The listing builds one solid part. Answer for the finished solid, in the listing's coordinates (mm). A direction names the side the tool comes from. Round coordinates to 2 decimals unless told otherwise and drop trailing zeros. Write each loop counter-clockwise with the first axis right and the second up, starting at its lowest first coordinate (ties: lowest second). Pieces come first, ordered by that corner, then holes. Notation, with made-up numbers: (48, 15.5) - (92, 15.5) arc R36 cw to (92, 49.5) - close; hole circle Ø2 at (-17, 85). An arc over 180 degrees is marked (long way). Return JSON: item names as keys, results as strings. Group by question number.
(1) Find the intervals of material crossed by line 1 along Y through (x, z) = (61.5, 58); line 2 along X through (y, z) = (19.45, 48); line 3 along Z through (x, y) = (61.75, 22.75), in increasing order. Write a range as [from, to].
(2) Determine the mould class of faces 4 (the flat face through (66, 17.5, 48)), 5 (the cylindrical face through (66.3, 19.27, 68.07)), 6 (the flat face through (55, 17, 72)) for opening direction X: +X half, -X half, draft (parallel to the pull), parting line (faces both ways), or undercut.
(3) Section C-C, the plane x = 54.25 is taken. Write down the section's boundary in (y, z), then the cut area to 3 significant figures.
(4) Each of these flat-tipped pins is pushed along its axis until it touches: pin 1 (4 mm diameter, centred on y = 15, z = 44.5, fed in from -X); pin 2 (8 mm diameter, centred on x = 61, y = 30.5, fed in from -Z); pin 3 (4.5 mm diameter, centred on x = 68, z = 49, fed in from -Y). Where does it stop, or does it pass through?
(5) Section D-D, the plane y = 31.75 is taken. Write down the section's boundary in (x, z).
(6) Section A-A, the plane y = 29 is taken. Write down the section's boundary in (x, z), then the cut area to 3 significant figures.
(7) Which of the six approach directions +Z, -Z, +X, -X, +Y, -Y give full straight-line access (tool end or side, diameter ignored) to faces 1 (the cylindrical face through (62.5, 27.145, 56.817)), 2 (the cylindrical face through (63.14, 27.1, 47.48)), 3 (the cylindrical face through (58.017, 24.76, 47.521))?
(8) Section B-B, the plane z = 59 is taken. Write down the section's boundary in (x, y), then the cut area to 3 significant figures.
```python
from build123d import *

# Parameters (mm, degrees)
BOX001027045206_W       = 8
BOX001027045206_H       = 6
BOX001027045206_DEPTH   = 10
CYLINDER272_R           = 2.2
CYLINDER272_DEPTH       = 30
CYLINDER271_R           = 2.2
CYLINDER271_DEPTH       = 30
CYLINDER271_PITCH_ANGLE = 90
CYLINDER270_R           = 1.7
CYLINDER270_DEPTH       = 30
CYLINDER270_PITCH_ANGLE = 90
BOX001027045200_W       = 10
BOX001027045200_H       = 9
BOX001027045200_DEPTH   = 10
CHAMFER015_SIZE         = 2
CHAMFER016_SIZE         = 2
FILLET046_R             = 3
CYLINDER045_R           = 1.9
CYLINDER045_DEPTH       = 200
BOX030_W                = 5.5
BOX030_H                = 10
BOX030_DEPTH            = 2.5
CYLINDER048_R           = 5.5
CYLINDER048_DEPTH       = 10
CYLINDER048_ROLL_ANGLE  = 90
CYLINDER050_R           = 5.5
CYLINDER050_DEPTH       = 10
CYLINDER050_ROLL_ANGLE  = 90
CYLINDER052_R           = 1.7
CYLINDER052_DEPTH       = 30
CYLINDER052_ROLL_ANGLE  = 90
CYLINDER053_R           = 1.7
CYLINDER053_DEPTH       = 30
CYLINDER053_ROLL_ANGLE  = 90
CYLINDER054_R           = 1.7
CYLINDER054_DEPTH       = 30
CYLINDER054_ROLL_ANGLE  = 90
CYLINDER047_R           = 5.5
CYLINDER047_DEPTH       = 10
CYLINDER047_ROLL_ANGLE  = 90
CYLINDER049_R           = 3
CYLINDER049_DEPTH       = 10
CYLINDER049_ROLL_ANGLE  = 90
CYLINDER051_R           = 3
CYLINDER051_DEPTH       = 10
CYLINDER051_ROLL_ANGLE  = 90
CYLINDER046_R           = 3
CYLINDER046_DEPTH       = 10
CYLINDER046_ROLL_ANGLE  = 90
BOX028_W                = 13
BOX028_H                = 8.5
BOX028_DEPTH            = 40
CHAMFER006_SIZE         = 2.5
CYLINDER273_R           = 2
CYLINDER273_DEPTH       = 10
CYLINDER273_PITCH_ANGLE = 90
BOX001027045201_W       = 3
BOX001027045201_H       = 8
BOX001027045201_DEPTH   = 8
FILLET047_R             = 3
CUT247_PITCH_ANGLE      = 90
CUT247_PLACEMENT_ANGLE  = 90


with BuildPart() as cube252:
    # Box001027045206 → Box001027045206 (new body)
    with BuildSketch(Plane(origin=(59.1, 20, 53), x_dir=(1, 0, 0), z_dir=(0, 0, 1))):
        with Locations((4, 3)):
            Rectangle(BOX001027045206_W, BOX001027045206_H)
    extrude(amount=BOX001027045206_DEPTH)


with BuildPart() as cylinder288:
    # Cylinder272 → Cylinder272 (new body)
    with BuildSketch(Plane(origin=(79.5, 5, 48), x_dir=(1, 0, 0), z_dir=(0, 0, 1))):
        Circle(CYLINDER272_R)
    extrude(amount=CYLINDER272_DEPTH)


with BuildPart() as cylinder287:
    # Cylinder271 → Cylinder271 (new body)
    with BuildSketch(Plane.XY):
        Circle(CYLINDER271_R)
    extrude(amount=CYLINDER271_DEPTH)


with BuildPart() as cylinder287_1:
    # Cylinder271 pitch: moved
    add(cylinder287.part.rotate(Axis((0, 0, 0), (0, 1, 0)), CYLINDER271_PITCH_ANGLE))


with BuildPart() as cylinder287_2:
    # Cylinder271 placement: moved
    add(cylinder287_1.part.moved(Location((74, 5, 58))))


with BuildPart() as cylinder286:
    # Cylinder270 → Cylinder270 (new body)
    with BuildSketch(Plane.XY):
        Circle(CYLINDER270_R)
    extrude(amount=CYLINDER270_DEPTH)


with BuildPart() as cylinder286_1:
    # Cylinder270 pitch: moved
    add(cylinder286.part.rotate(Axis((0, 0, 0), (0, 1, 0)), CYLINDER270_PITCH_ANGLE))


with BuildPart() as cylinder286_2:
    # Cylinder270 placement: moved
    add(cylinder286_1.part.moved(Location((57, 5, 58))))


with BuildPart() as led_pt_holder001:
    # Box001027045200 → Box001027045200 (new body)
    with BuildSketch(Plane(origin=(71, 1, 53), x_dir=(1, 0, 0), z_dir=(0, 0, 1))):
        with Locations((5, 4.5)):
            Rectangle(BOX001027045200_W, BOX001027045200_H)
    extrude(amount=BOX001027045200_DEPTH)

    # Chamfer015
    chamfer015_edges = [led_pt_holder001.edges().sort_by_distance(p)[0] for p in [
        (71, 10, 58),
    ]]
    chamfer(chamfer015_edges, length=CHAMFER015_SIZE)


with BuildPart() as led_pt_holder001_1:
    # Chamfer015 placement: moved
    add(led_pt_holder001.part.moved(Location((-1.5, 0, 0))))

    # Chamfer016
    chamfer016_edges = [led_pt_holder001_1.edges().sort_by_distance(p)[0] for p in [
        (69.5, 4.5, 63),
        (69.5, 4.5, 53),
    ]]
    chamfer(chamfer016_edges, length=CHAMFER016_SIZE)

    # Cut242: cut Cylinder286
    add(cylinder286_2.part, mode=Mode.SUBTRACT)

    # Cut243: cut Cylinder287
    add(cylinder287_2.part, mode=Mode.SUBTRACT)

    # Fillet046
    fillet046_edges = [led_pt_holder001_1.edges().sort_by_distance(p)[0] for p in [
        (69.5, 4.5, 55),
        (69.5, 4.5, 61),
    ]]
    fillet(fillet046_edges, radius=FILLET046_R)

    # Cut245: cut Cylinder288
    add(cylinder288.part, mode=Mode.SUBTRACT)


with BuildPart() as part_mirroring015:
    # Part__Mirroring015: instance of led-pt-holder001
    add(led_pt_holder001_1.part.mirror(Plane(origin=(60, 0, 0), x_dir=(0, -1, 0), z_dir=(1, 0, 0))))


with BuildPart() as part_mirroring015_1:
    # Part__Mirroring015 placement: moved
    add(part_mirroring015.part.moved(Location((18.6, 0, 0))))


with BuildPart() as pt_holder:
    # Part__Mirroring019: instance of Part__Mirroring015
    add(part_mirroring015_1.part.mirror(Plane(origin=(0, 0, 0), x_dir=(1, 0, 0), z_dir=(0, 1, 0))))


with BuildPart() as pt_holder_1:
    # Part__Mirroring019 placement: moved
    add(pt_holder.part.moved(Location((0, 34, 0))))

    # Fusion112161: union Cube252
    add(cube252.part)


with BuildPart() as m3_studding004:
    # Cylinder045 → Cylinder045 (new body)
    with BuildSketch(Plane(origin=(61.5, 15, 2), x_dir=(1, 0, 0), z_dir=(0, 0, 1))):
        Circle(CYLINDER045_R)
    extrude(amount=CYLINDER045_DEPTH)


with BuildPart() as m3_nut_hole:
    # Box030 → Box030 (new body)
    with BuildSketch(Plane(origin=(59, 11.7, 74), x_dir=(1, 0, 0), z_dir=(0, 0, 1))):
        with Locations((2.75, 5)):
            Rectangle(BOX030_W, BOX030_H)
    extrude(amount=BOX030_DEPTH)


with BuildPart() as cylinder088:
    # Cylinder048 → Cylinder048 (new body)
    with BuildSketch(Plane.XY):
        Circle(CYLINDER048_R)
    extrude(amount=CYLINDER048_DEPTH)


with BuildPart() as cylinder088_1:
    # Cylinder048 roll: moved
    add(cylinder088.part.rotate(Axis((0, 0, 0), (1, 0, 0)), CYLINDER048_ROLL_ANGLE))


with BuildPart() as cylinder088_2:
    # Cylinder048 placement: moved
    add(cylinder088_1.part.moved(Location((68, 17.5, 68))))


with BuildPart() as cylinder090:
    # Cylinder050 → Cylinder050 (new body)
    with BuildSketch(Plane.XY):
        Circle(CYLINDER050_R)
    extrude(amount=CYLINDER050_DEPTH)


with BuildPart() as cylinder090_1:
    # Cylinder050 roll: moved
    add(cylinder090.part.rotate(Axis((0, 0, 0), (1, 0, 0)), CYLINDER050_ROLL_ANGLE))


with BuildPart() as cylinder090_2:
    # Cylinder050 placement: moved
    add(cylinder090_1.part.moved(Location((68, 17.5, 48))))


with BuildPart() as cylinder092:
    # Cylinder052 → Cylinder052 (new body)
    with BuildSketch(Plane.XY):
        Circle(CYLINDER052_R)
    extrude(amount=CYLINDER052_DEPTH)


with BuildPart() as cylinder092_1:
    # Cylinder052 roll: moved
    add(cylinder092.part.rotate(Axis((0, 0, 0), (1, 0, 0)), CYLINDER052_ROLL_ANGLE))


with BuildPart() as cylinder092_2:
    # Cylinder052 placement: moved
    add(cylinder092_1.part.moved(Location((68, 26, 48))))


with BuildPart() as cylinder052:
    # Cylinder053 → Cylinder053 (new body)
    with BuildSketch(Plane.XY):
        Circle(CYLINDER053_R)
    extrude(amount=CYLINDER053_DEPTH)


with BuildPart() as cylinder052_1:
    # Cylinder053 roll: moved
    add(cylinder052.part.rotate(Axis((0, 0, 0), (1, 0, 0)), CYLINDER053_ROLL_ANGLE))


with BuildPart() as cylinder052_2:
    # Cylinder053 placement: moved
    add(cylinder052_1.part.moved(Location((68, 27, 68))))


with BuildPart() as cylinder093:
    # Cylinder054 → Cylinder054 (new body)
    with BuildSketch(Plane.XY):
        Circle(CYLINDER054_R)
    extrude(amount=CYLINDER054_DEPTH)


with BuildPart() as cylinder093_1:
    # Cylinder054 roll: moved
    add(cylinder093.part.rotate(Axis((0, 0, 0), (1, 0, 0)), CYLINDER054_ROLL_ANGLE))


with BuildPart() as cylinder093_2:
    # Cylinder054 placement: moved
    add(cylinder093_1.part.moved(Location((55, 26, 58))))


with BuildPart() as trolley_clearances_and_screws:
    # Cylinder047 → Cylinder047 (new body)
    with BuildSketch(Plane.XY):
        Circle(CYLINDER047_R)
    extrude(amount=CYLINDER047_DEPTH)


with BuildPart() as trolley_clearances_and_screws_1:
    # Cylinder047 roll: moved
    add(trolley_clearances_and_screws.part.rotate(Axis((0, 0, 0), (1, 0, 0)), CYLINDER047_ROLL_ANGLE))


with BuildPart() as trolley_clearances_and_screws_2:
    # Cylinder047 placement: moved
    add(trolley_clearances_and_screws_1.part.moved(Location((55, 17.5, 58))))

    # Fusion028: union Cylinder088, Cylinder090, Cylinder092, Cylinder052, Cylinder093
    add(cylinder088_2.part)
    add(cylinder090_2.part)
    add(cylinder092_2.part)
    add(cylinder052_2.part)
    add(cylinder093_2.part)


with BuildPart() as cylinder089:
    # Cylinder049 → Cylinder049 (new body)
    with BuildSketch(Plane.XY):
        Circle(CYLINDER049_R)
    extrude(amount=CYLINDER049_DEPTH)


with BuildPart() as cylinder089_1:
    # Cylinder049 roll: moved
    add(cylinder089.part.rotate(Axis((0, 0, 0), (1, 0, 0)), CYLINDER049_ROLL_ANGLE))


with BuildPart() as cylinder089_2:
    # Cylinder049 placement: moved
    add(cylinder089_1.part.moved(Location((68, 21, 68))))


with BuildPart() as cylinder091:
    # Cylinder051 → Cylinder051 (new body)
    with BuildSketch(Plane.XY):
        Circle(CYLINDER051_R)
    extrude(amount=CYLINDER051_DEPTH)


with BuildPart() as cylinder091_1:
    # Cylinder051 roll: moved
    add(cylinder091.part.rotate(Axis((0, 0, 0), (1, 0, 0)), CYLINDER051_ROLL_ANGLE))


with BuildPart() as cylinder091_2:
    # Cylinder051 placement: moved
    add(cylinder091_1.part.moved(Location((68, 21, 48))))


with BuildPart() as trolley_hubs:
    # Cylinder046 → Cylinder046 (new body)
    with BuildSketch(Plane.XY):
        Circle(CYLINDER046_R)
    extrude(amount=CYLINDER046_DEPTH)


with BuildPart() as trolley_hubs_1:
    # Cylinder046 roll: moved
    add(trolley_hubs.part.rotate(Axis((0, 0, 0), (1, 0, 0)), CYLINDER046_ROLL_ANGLE))


with BuildPart() as trolley_hubs_2:
    # Cylinder046 placement: moved
    add(trolley_hubs_1.part.moved(Location((55, 21, 58))))

    # Fusion027: union Cylinder089, Cylinder091
    add(cylinder089_2.part)
    add(cylinder091_2.part)


with BuildPart() as trolley_b001:
    # Box028 → Box028 (new body)
    with BuildSketch(Plane(origin=(55, 12.5, 41), x_dir=(1, 0, 0), z_dir=(0, 0, 1))):
        with Locations((6.5, 4.25)):
            Rectangle(BOX028_W, BOX028_H)
    extrude(amount=BOX028_DEPTH)

    # Fusion029: union trolley-hubs
    add(trolley_hubs_2.part)

    # Cut017: cut trolley-clearances-and-screws
    add(trolley_clearances_and_screws_2.part, mode=Mode.SUBTRACT)

    # Cut019: cut M3-nut-hole
    add(m3_nut_hole.part, mode=Mode.SUBTRACT)

    # Chamfer006
    chamfer006_edges = [trolley_b001.edges().sort_by_distance(p)[0] for p in [
        (55, 19.25, 55),
        (68, 19.25, 45),
        (55, 19.25, 61),
        (68, 19.25, 65),
        (68, 19.25, 51),
        (68, 19.25, 71),
    ]]
    chamfer(chamfer006_edges, length=CHAMFER006_SIZE)

    # Cut033: cut m3-studding004
    add(m3_studding004.part, mode=Mode.SUBTRACT)


with BuildPart() as cylinder289:
    # Cylinder273 → Cylinder273 (new body)
    with BuildSketch(Plane.XY):
        Circle(CYLINDER273_R)
    extrude(amount=CYLINDER273_DEPTH)


with BuildPart() as cylinder289_1:
    # Cylinder273 pitch: moved
    add(cylinder289.part.rotate(Axis((0, 0, 0), (0, 1, 0)), CYLINDER273_PITCH_ANGLE))


with BuildPart() as cylinder289_2:
    # Cylinder273 placement: moved
    add(cylinder289_1.part.moved(Location((-3, 4, 4.5))))


with BuildPart() as trolley:
    # Box001027045201 → Box001027045201 (new body)
    with BuildSketch(Plane.XY):
        with Locations((1.5, 4)):
            Rectangle(BOX001027045201_W, BOX001027045201_H)
    extrude(amount=BOX001027045201_DEPTH)

    # Fillet047
    fillet047_edges = [trolley.edges().sort_by_distance(p)[0] for p in [
        (1.5, 0, 8),
        (1.5, 8, 8),
    ]]
    fillet(fillet047_edges, radius=FILLET047_R)

    # Cut247: cut Cylinder289
    add(cylinder289_2.part, mode=Mode.SUBTRACT)


with BuildPart() as trolley_1:
    # Cut247 pitch: moved
    add(trolley.part.rotate(Axis((0, 0, 0), (0, 1, 0)), CUT247_PITCH_ANGLE))


with BuildPart() as trolley_2:
    # Cut247 placement: moved
    add(trolley_1.part.moved(Location((64, 20, 49))).rotate(Axis((64, 20, 49), (0, 0, 1)), CUT247_PLACEMENT_ANGLE))

    # Fusion112159: union trolley-b001
    add(trolley_b001.part)

    # Fusion112164: union pt-holder
    add(pt_holder_1.part)


solid = trolley_2.part
```
Working result:
{
 "1": {"line 1": "y = [12.5, 13.1], [16.9, 26.8], [31.2, 33]", "line 2": "x = [55, 66.3], [69.7, 71]", "line 3": "z = [46, 49], [53, 63]"},
 "2": {"face 4": "draft", "face 5": "undercut", "face 6": "-X half"},
 "3": {"outline": "(17.5, 53.67) - (21, 53.67) - (21, 56.47) - (17.5, 56.47) - close; (17.5, 59.53) - (21, 59.53) - (21, 62.33) - (17.5, 62.33) - close", "area": "19.6 mm^2"},
 "4": {"pin 1": "stops at x = 55", "pin 2": "stops at z = 46", "pin 3": "stops at y = 17.5"},
 "5": {"outline": "(59.1, 53) - (67.1, 53) - (68.22, 54.12) arc R3 ccw to (69.1, 56.24) - (69.1, 59.76) arc R3 ccw to (68.22, 61.88) - (67.1, 63) - (59.1, 63) - close"},
 "6": {"outline": "(61.3, 53) - (67.1, 53) - (68.22, 54.12) arc R3 ccw to (69.1, 56.24) - (69.1, 56.3) - (64.6, 56.3) - (64.6, 55.8) - (61.3, 55.8) - close; (61.3, 60.2) - (64.6, 60.2) - (64.6, 59.7) - (69.1, 59.7) - (69.1, 59.76) arc R3 ccw to (68.22, 61.88) - (67.1, 63) - (61.3, 63) - close", "area": "43.8 mm^2"},
 "7": {"face 1": "-X", "face 2": "-Z, +X, +Y", "face 3": "-Z"},
 "8": {"outline": "(52.17, 17.5) - (53.63, 17.5) - (53.63, 21) - (52.17, 21) - close; (56.37, 17.5) - (60.41, 17.5) - (60.41, 16.56) arc R1.9 cw (long way) to (60.41, 13.44) - (60.41, 12.5) - (68, 12.5) - (68, 21) - (67.1, 21) - (67.1, 24) - (69.1, 26) - (69.1, 27.63) - (64.6, 27.63) - (64.6, 27.04) - (60.1, 27.04) arc R2.2 cw to (59.1, 26.8) - (59.1, 21) - (56.37, 21) - close; (59.1, 31.2) arc R2.2 cw to (60.1, 30.96) - (64.6, 30.96) - (64.6, 30.37) - (69.1, 30.37) - (69.1, 33) - (59.1, 33) - close", "area": "152 mm^2"}
}
